Source: CAD feature listing. Evaluate the final solid. Frame: model axes, mm. A direction names the side the tool comes from. Give positions to 0.01 mm unless a question says otherwise; leave off trailing zeros. Write each loop counter-clockwise with the first axis right and the second up, starting at its lowest first coordinate (ties: lowest second). Pieces come first, ordered by that corner, then holes. Notation, with made-up numbers: (-38, -23.5) -> (-24, -23.5) arc R16 cw to (-24, -15.5) -> close; hole circle Ø7 at (-2, 12). An arc over 180 degrees is marked (long way). Answer as a JSON object with one key per item and string values. Group by question number.
Item 1: Pull-direction query (X, two-part tool) for faces 6 (the face through (-7.47, 14, 1.57)), 7 (the face through (4.613, 15.183, 1.565)), 8 (the face through (-6.32, 13.5, 1.61)); classes: pulls with the +X half, pulls with the -X half, needs draft (parallel to the pull), parting line crosses it, or undercut.
Item 2: Section query A-A on y = -6. Return the cut outline in (x, z) (3 decimals), plus the area to 3 significant figures.
Item 3: Access query for faces 1 (the face through (-14.45, 3.55, 1.61)), 2 (the face through (-3.57, 14.48, 1.61)), 3 (the face through (10.055, 11.01, 1.61)), 4 (the face through (12.01, 8.84, 1.61)), 5 (the face through (2.25, -14.71, 1.61)). Directions: +Z, -Z, +X, -X, +Y, -Y. A direction counts if a zero-diameter tool reaches every point of the face in a straight line with its end or side. Return the directions, or none.
Item 4: Ray query, probe 1 along X at (y, z) = (0, 1.25); probe 2 along X at (y, z) = (10, 1.2); probe 3 along Y at (x, z) = (0, 1.35). Return the intervals inside material, ascending. Write a range as from..to.
from build123d import *

# Parameters (mm, degrees)
F0_R            = 15.8688012495
F1_DEPTH        = 3.175
F3_DEPTH        = 3.175
F3_COPIES_COUNT = 32


# Not quite as in the source:
# - a pattern or mirror of a feature is missing from the dataset's text; its kind, count and spacing are read off the source's solid


with BuildPart() as f1:
    # F0 (on Top) → F1 (new body)
    with BuildSketch(Plane.XY):
        Circle(F0_R)
        with BuildLine():
            ThreePointArc((3.0120159229, 0.8763), (0, -3.1369), (-3.0120159229, 0.8763))
            Line((-3.0120159229, 0.8763), (3.0120159229, 0.8763))
        make_face(mode=Mode.SUBTRACT)
    extrude(amount=F1_DEPTH)

    # F2 (on face) → F3 (cut, through all)
    with BuildSketch(Plane.XY.offset(3.175)):
        with BuildLine():
            Line((-13.9312413972, 0.274735453), (-15.8329891451, 1.065508248))
            ThreePointArc((-15.8329891451, 1.065508248), (-15.8688012495, 0), (-15.8329891451, -1.065508248))
            Line((-15.8329891451, -1.065508248), (-13.9312413972, -0.274735453))
            ThreePointArc((-13.9312413972, -0.274735453), (-13.747940143, 0), (-13.9312413972, 0.274735453))
        make_face()
    f3 = extrude(amount=-F3_DEPTH, mode=Mode.SUBTRACT)

    # F3_copies: F3 ×32 about axis
    f3_copies_axis = Axis((0, 0, 0), (0, 0, 1))
    for i in range(1, F3_COPIES_COUNT):
        add(f3.rotate(f3_copies_axis, i * 360 / F3_COPIES_COUNT), mode=Mode.SUBTRACT)


solid = f1.part
Worked answers:
{
 "1": {"face 6": "pulls with the -X half", "face 7": "pulls with the +X half", "face 8": "undercut"},
 "2": {"outline": "(-13.179, 0) -> (13.179, 0) -> (13.179, 3.175) -> (-13.179, 3.175) -> close", "area": "83.7 mm^2"},
 "3": {"face 1": "+Z, -Z, -X", "face 2": "+Z, -Z, +Y", "face 3": "+Z, -Z", "face 4": "+Z, -Z, +X", "face 5": "+Z, -Z, -Y"},
 "4": {"probe 1": "-13.75..-3.14, 3.14..13.75", "probe 2": "-12.32..-10.88, -9.64..9.64, 10.88..12.32", "probe 3": "-13.75..-3.14, 0.88..13.75"}
}
